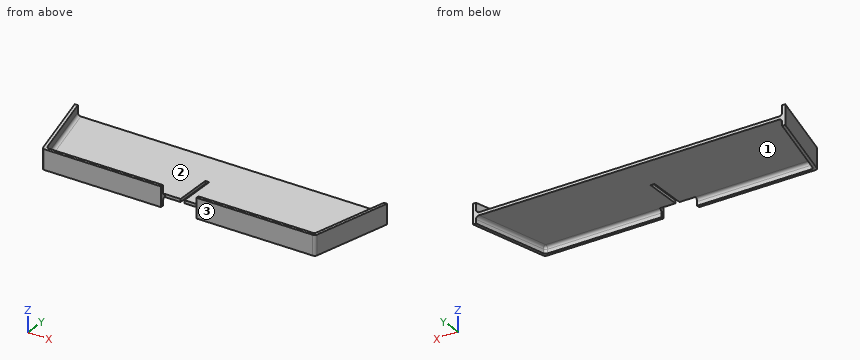
```python
from build123d import *

# Parameters (mm, degrees)
BOSS_EXTRUDE2_DEPTH            = 1.5
BOSS_EXTRUDE3_DEPTH            = 5
BOSS_EXTRUDE3_DEPTH_BACK       = 5
FILLET1_R                      = 1.5
CUT_EXTRUDE1_REACH             = 7
SKETCH6_W                      = 8
SKETCH6_H                      = 3
CUT_EXTRUDE1_DIRECTION_2_DEPTH = 6


with BuildPart() as part:
    # Sketch1 → Boss-Extrude2 (new body)
    with BuildSketch(Plane.XY):
        Polygon((0, 0), (158, 0), (148, -40), (80, -40), (80, -18), (78, -18), (78, -40), (10, -40), align=None)
    extrude(amount=BOSS_EXTRUDE2_DEPTH)

    # Sketch5 → Boss-Extrude3 (add, two sides)
    with BuildSketch(Plane.XY.offset(1.5)) as boss_extrude3_sk:
        Polygon((156.45383539, 0), (158, 0), (148, -40), (88, -40), (88, -38.5), (146.82883539, -38.5), align=None)
        Polygon((70, -38.5), (70, -40), (10, -40), (0, 0), (1.54616461, 0), (11.17116461, -38.5), align=None)
    extrude(amount=BOSS_EXTRUDE3_DEPTH)
    extrude(boss_extrude3_sk.sketch, amount=-BOSS_EXTRUDE3_DEPTH_BACK)

    # Fillet1
    fillet1_edges = [part.edges().sort_by_distance(p)[0] for p in [
        (148, -40, 1.5),
        (10, -40, 1.5),
        (151.64133539, -19.25, 0),
        (117.414417695, -38.5, 0),
        (146.82883539, -38.5, -1.75),
        (117.414417695, -38.5, 1.5),
        (151.64133539, -19.25, 1.5),
        (146.82883539, -38.5, 4),
        (40.585582305, -38.5, 0),
        (6.35866461, -19.25, 0),
        (11.17116461, -38.5, -1.75),
        (6.35866461, -19.25, 1.5),
        (40.585582305, -38.5, 1.5),
        (11.17116461, -38.5, 4),
    ]]
    fillet(fillet1_edges, radius=FILLET1_R)

    # Sketch6 → Cut-Extrude1 (cut, up to next)
    with BuildSketch(Plane.XY.offset(1.5), mode=Mode.PRIVATE) as cut_extrude1_sk1:
        with Locations((74, -38.5)):
            Rectangle(SKETCH6_W, SKETCH6_H)
    cut_extrude1_tool1 = extrude(cut_extrude1_sk1.sketch, amount=-CUT_EXTRUDE1_REACH, mode=Mode.PRIVATE) & part.part
    add(cut_extrude1_tool1.solids().sort_by_distance((74, -38.5, 1.5))[0], mode=Mode.SUBTRACT)
    # Sketch6 → Cut-Extrude1 (cut, up to next)
    with BuildSketch(Plane.XY.offset(1.5), mode=Mode.PRIVATE) as cut_extrude1_sk2:
        with Locations((84, -38.5)):
            Rectangle(SKETCH6_W, SKETCH6_H)
    cut_extrude1_tool2 = extrude(cut_extrude1_sk2.sketch, amount=-CUT_EXTRUDE1_REACH, mode=Mode.PRIVATE) & part.part
    add(cut_extrude1_tool2.solids().sort_by_distance((84, -38.5, 1.5))[0], mode=Mode.SUBTRACT)

    # Sketch6 → Cut-Extrude1 direction 2 (cut)
    with BuildSketch(Plane.XY.offset(1.5)):
        with Locations((74, -38.5)):
            Rectangle(SKETCH6_W, SKETCH6_H)
        with Locations((84, -38.5)):
            Rectangle(SKETCH6_W, SKETCH6_H)
    extrude(amount=CUT_EXTRUDE1_DIRECTION_2_DEPTH, mode=Mode.SUBTRACT)


solid = part.part
```
CAD build for the part. Positions are in the model's coordinates, mm. Face numbers are marked on the shaded views. A direction names the side the tool comes from. Round coordinates to 2 decimals unless told otherwise and drop trailing zeros. Loops run counter-clockwise (first coordinate to the right, second up) from the corner with the lowest first, then second, coordinate; pieces in that order, holes last. Notation, with made-up numbers: (15, 27) - (70, 27) arc R8 cw to (70, 32) - close; hole circle Ø8 at (-1.5, -11.5). An arc over 180 degrees is marked (long way). Return JSON: item names as keys, results as strings. Group by question number.
Q1. Band-saw the part on A-A on z = 4.5. Give the cut face in (x, y).
Q2. Flat gauge pins, fed straight in: pin 1 Ø3 at (x, z) = (44.5, 4.5) entering from +Y; pin 2 Ø1.5 at (x, y) = (61, -18) entering from +Z; pin 3 Ø12 at (x, y) = (81.5, -18.5) entering from -Z. Where does each tip first touch, or does it go through?
Q3. Band-saw the part on B-B on x = 47.5. Give the cut face in (y, z).
Q4. Drill centre lines: line 1 along Y through (x, z) = (106, 3.25); line 2 along X through (y, z) = (-37, 2.75); line 3 along Z through (x, y) = (139.5, -20.5). Where is each one in solid material? Low to high. Write a range as [from, to].
Q5. Tool access for the marked faces 1, 2 and 3: list every direction of +Z, -Z, +X, -X, +Y, -Y with a clear straight run to the whole face (end or side of a thin tool).
Solutions:
{
 "1": {"outline": "(0, 0) - (9.72, -38.86) arc R1.5 ccw to (11.17, -40) - (70, -40) - (70, -38.5) - (12.34, -38.5) arc R1.5 cw to (10.89, -37.36) - (1.55, 0) - close; (88, -40) - (146.83, -40) arc R1.5 ccw to (148.28, -38.86) - (158, 0) - (156.45, 0) - (147.11, -37.36) arc R1.5 cw to (145.66, -38.5) - (88, -38.5) - close"},
 "2": {"pin 1": "stops at y = -38.5", "pin 2": "stops at z = 1.5", "pin 3": "stops at z = 0"},
 "3": {"outline": "(-40, -3.5) - (-38.5, -3.5) - (-38.5, -1.5) arc R1.5 cw to (-37, 0) - (0, 0) - (0, 1.5) - (-37, 1.5) arc R1.5 cw to (-38.5, 3) - (-38.5, 6.5) - (-40, 6.5) - close"},
 "4": {"line 1": "y = [-40, -38.5]", "line 2": "x = [9.25, 10.82], [147.18, 148.75]", "line 3": "z = [0, 1.5]"},
 "5": {"face 1": "-Z, +Y", "face 2": "+Z, +Y", "face 3": "+Z, -Z, +X, -X, -Y"}
}
